Could you check a few things on this model? Use its own coordinates, in mm. A direction names the side the tool comes from. Round coordinates to 2 decimals unless told otherwise and drop trailing zeros. Loops run counter-clockwise (first coordinate to the right, second up) from the corner with the lowest first, then second, coordinate; pieces in that order, holes last.
from build123d import *

# Parameters (mm, degrees)
F0_W     = 96.6246202588
F0_H     = 64.4804909825
F1_DEPTH = 12.7
F2_R     = 39.0357793673
F3_DEPTH = 50.8
F4_R     = 28.6832588226
F5_DEPTH = 94.996
F7_DEPTH = 38.1
F9_DEPTH = 72.898


with BuildPart() as f1:
    # F0 (on Top) → F1 (new body)
    with BuildSketch(Plane.XY):
        Rectangle(F0_W, F0_H)
    extrude(amount=F1_DEPTH)

    # F2 (on Top) → F3 (join)
    with BuildSketch(Plane.XY):
        with Locations((70.9010735154, 0)):
            Circle(F2_R)
    extrude(amount=F3_DEPTH)

    # F4 (on face) → F5 (cut)
    with BuildSketch(Plane.XY.offset(50.8)):
        with Locations((70.9010735154, 0)):
            Circle(F4_R)
    extrude(amount=-F5_DEPTH, mode=Mode.SUBTRACT)

    # F6 (on face) → F7 (join)
    with BuildSketch(Plane.XY.offset(12.7)):
        with BuildLine():
            Line((33.3239030226, 10.5711081997), (-34.8241180182, 10.5711081997))
            Line((-34.8241180182, 10.5711081997), (-34.8241180182, -10.5711081997))
            Line((-34.8241180182, -10.5711081997), (33.3239030226, -10.5711081997))
            ThreePointArc((33.3239030226, -10.5711081997), (31.8652941481, 0), (33.3239030226, 10.5711081997))
        make_face()
    extrude(amount=F7_DEPTH)

    # F8 (on face) → F9 (cut)
    with BuildSketch(Plane.XZ.offset(10.5711081997)):
        Polygon((-34.8241180182, 12.7), (33.3239030226, 50.8), (-34.8241180182, 50.8), align=None)
    extrude(amount=-F9_DEPTH, mode=Mode.SUBTRACT)


solid = f1.part
Item 1: If we section it at B-B, the plane x = 93.5: Please give me the cut outline in (y, z), then the cut area to 3 significant figures.
Results list:
outline: (-31.83, 0) - (-17.66, 0) - (-17.66, 50.8) - (-31.83, 50.8) - close; (17.66, 0) - (31.83, 0) - (31.83, 50.8) - (17.66, 50.8) - close
area: 1,440 mm2
Item 2: For faces 4 (the flat face through (-1, -32.24, 6)), 5 (the flat face through (-11, 15, 12.7)), 6 (the flat face through (14, -10.571, 23)), 7 (the cylindrical face through (109.905, -1.567, 25.044)), which set-ups out of +Z, -Z, +X, -X, +Y, -Y let a thin tool reach every point of the face, with its end or its side?
Results list:
face 4: +Z, -Z, -X, -Y
face 5: +Z, -X
face 6: +Z, -X, -Y
face 7: +Z
Item 3: If we section it at A-A, the plane y = 0: Please give me the cut outline in (x, z), then the cut area to 3 significant figures.
Results list:
outline: (-48.31, 0) - (42.22, 0) - (42.22, 50.8) - (33.32, 50.8) - (-34.82, 12.7) - (-48.31, 12.7) - close; (99.58, 0) - (109.94, 0) - (109.94, 50.8) - (99.58, 50.8) - close
area: 3,310 mm2
Item 4: If we section it at D-D, the plane y = 14.5: Please give me the cut outline in (x, z), then the cut area to 3 significant figures.
Results list:
outline: (-48.31, 0) - (46.15, 0) - (46.15, 50.8) - (34.66, 50.8) - (34.66, 12.7) - (-48.31, 12.7) - close; (95.65, 0) - (107.14, 0) - (107.14, 50.8) - (95.65, 50.8) - close
area: 2,220 mm2
Item 5: We'd pull the mould along X, two halves only. Please class faces 1 (the flat face through (-1.2, -0.1, 31.5)), 2 (the flat face through (12, 1, 0)), 3 (the cylindrical face through (98.26, 8.62, 25.76)): released by +X, released by -X, zero draft, split by the parting line, or undercut.
Results list:
face 1: released by -X
face 2: zero draft
face 3: undercut
Item 6: If I drill on line 1 along Y through (x, z) = (72, 21.5); line 2 along X through (y, z) = (0.5, 38); line 3 along Y through (x, z) = (-1.5, 30.5), over which ranges is the centre line in solid material (lowest first)?
Results list:
line 1: y = -39.02 to -28.66, 28.66 to 39.02
line 2: x = 10.43 to 42.22, 99.58 to 109.93
line 3: y = -10.57 to 10.57
Item 7: If we section it at C-C, the plane z = 22: Please give me the cut outline in (x, y), then the cut area to 3 significant figures.
Results list:
outline: (-18.19, -10.57) - (33.32, -10.57) arc R39.04 ccw (long way) to (33.32, 10.57) - (-18.19, 10.57) - close; hole circle Ø57.37 at (70.9, 0)
area: 3,270 mm2
Item 8: Will these pins go through, and if not, where does the flat tip stop? pin 1 (4 mm diameter, centred on x = -6, z = 9.5, fed in from -Y); pin 2 (5 mm diameter, centred on y = 22.5, z = 22.5, fed in from -X); pin 3 (11.5 mm diameter, centred on x = -7, z = 25.5, fed in from -Y); pin 4 (6 mm diameter, centred on x = -9.5, y = 2, fed in from -Z).
Results list:
pin 1: stops at y = -32.24
pin 2: stops at x = 37.38
pin 3: stops at y = -10.57
pin 4: stops at z = 0
